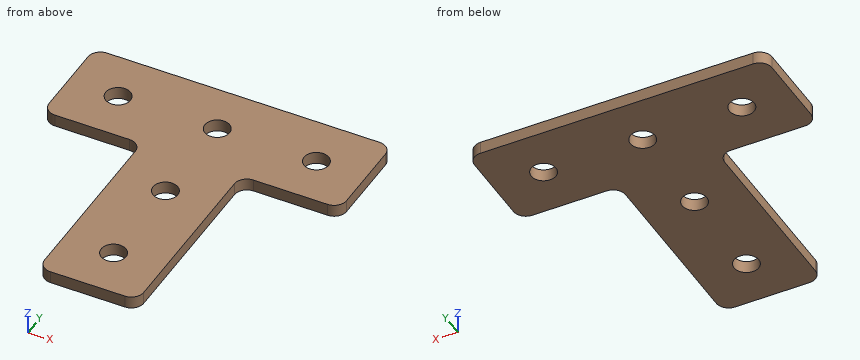
Autodesk Inventor part; units mm, degrees
ref_plane "YZ Plane" through (0, 0, 0) normal (1, 0, 0) x (0, 1, 0)
ref_plane "XZ Plane" through (0, 0, 0) normal (0, 1, 0) x (-1, 0, 0)
ref_plane "XY Plane" through (0, 0, 0) normal (0, 0, 1) x (1, 0, 0)
sketch "Sketch1" plane through (0, 0, 0) normal (0, 0, 1) x (1, 0, 0)
  line L0 (-18.0361, 37.9933) -> (2.0277, 37.9933)
  line L1 (6.0832, 12.5933) -> (6.0832, -38.2067)
  line L2 (6.0832, -38.2067) -> (-19.3168, -38.2067)
  line L3 (-19.3168, -38.2067) -> (-19.3168, 12.5933)
  line L4 (-44.7168, 37.9933) -> (31.4832, 37.9933)
  line L5 (31.4832, 37.9933) -> (31.4832, 12.5933)
  line L6 (-44.7168, 12.5933) -> (-44.7168, 37.9933)
  line L7 (31.4832, 12.5933) -> (6.0832, 12.5933)
  line L8 (-19.3168, 12.5933) -> (-44.7168, 12.5933)
  point P0 (0, 0)
  dimension "d0" = 76.2
  dimension "d1" = 25.4
  dimension "d2" = 25.4
  dimension "d3" = 25.4
  dimension "d4" = 50.8
  dimension "d5" = 25.4
extrude "Extrusion1" add sketch "Sketch1" along normal blind 3.175
fillet "Fillet1" radius 3.175 3 edges at (-44.7168, 12.5933, 1.5875) (-19.3168, 12.5933, 1.5875) (-19.3168, -38.2067, 1.5875)
fillet "Fillet2" radius 3.175 1 edges at (6.0832, -38.2067, 1.5875)
fillet "Fillet3" radius 3.175 3 edges at (6.0832, 12.5933, 1.5875) (31.4832, 12.5933, 1.5875) (31.4832, 37.9933, 1.5875)
fillet "Fillet4" radius 3.175 1 edges at (-44.7168, 37.9933, 1.5875)
sketch "Sketch2" plane through (0, 0, 3.175) normal (0, 0, 1) x (1, 0, 0)
  line L0 (31.4832, 15.7683) -> (31.4832, 34.8183)
  line L1 (31.4832, 25.2933) -> (-44.7168, 25.2933) construction
  line L2 (-44.7168, 34.8183) -> (-44.7168, 15.7683)
  line L3 (28.3082, 37.9933) -> (-41.5418, 37.9933)
  line L4 (-6.6168, 37.9933) -> (-6.6168, -38.2067) construction
  line L5 (-16.1418, -38.2067) -> (2.9082, -38.2067)
  circle A0 centre (18.7832, 25.2933) radius 3.175
  circle A1 centre (-6.6168, 25.2933) radius 3.175
  circle A2 centre (-32.0168, 25.2933) radius 3.175
  circle A3 centre (-6.6168, -0.1067) radius 3.175
  circle A4 centre (-6.6168, -25.5067) radius 3.175
  point P0 (0, 0)
  dimension "d12" = 6.35
  dimension "d13" = 12.7
  dimension "d16" = 25.4
  dimension "d23" = 25.4
extrude "Extrusion2" cut sketch "Sketch2" against normal through all
properties part number "Frame T Gussets"
The listing builds one solid part. Answer for the finished solid, in the listing's coordinates (mm). Coordinates: 2 decimals unless noted, no trailing zeros. Write each loop counter-clockwise with the first axis right and the second up, starting at its lowest first coordinate (ties: lowest second). Pieces come first, ordered by that corner, then holes. Notation, with made-up numbers: M -12,16 L 47,16 A33 ccw 47,51 Z; hole C 53,8 d1. An arc over 180 degrees is marked long. Use a Markdown table: item, result. Add a question column.
1. Given P1, Ø1.6, axis at y = -3.5, z = 2, coming from the +X side; P2, Ø8.5, axis at x = -6.62, y = -0.11, coming from the -Z side; P3, Ø1.6, axis at x = -34.5, z = 2, coming from the -Y side, each flat-ended and moving along its own axis, determine where each tip first touches the part or whether it passes through.
2. Section A-A (x = 11.5) is taken. Give the vertices of the cut face in (y, z) (3 decimals), plus the area to 3 significant figures.
3. Section B-B (y = -6) is taken. Give the vertices of the cut face in (x, z) (3 decimals).
4. Straight lines are drawn through the part: line 1 along X through (y, z) = (27, 1.1); line 2 along X through (y, z) = (7.5, 1.3); line 3 along Y through (x, z) = (11, 0.55). For each, find the intervals that lie inside material, in ascending order. Write a range as [from, to].
5. Section C-C (z = 1.3) is taken. Give the vertices of the cut face in (x, y) (3 decimals), plus the area to 3 significant figures.
Data:
| question | item | result |
|---|---|---|
| 1 | P1 | stops at x = 6.08 |
| 1 | P2 | stops at z = 0 |
| 1 | P3 | stops at y = 12.59 |
| 2 | outline | M 12.593,0 L 37.993,0 L 37.993,3.175 L 12.593,3.175 Z |
| 2 | area | 80.6 mm2 |
| 3 | outline | M -19.317,0 L 6.083,0 L 6.083,3.175 L -19.317,3.175 Z |
| 4 | line 1 | x = [-44.72, -34.69], [-29.34, -9.29], [-3.94, 16.11], [21.46, 31.48] |
| 4 | line 2 | x = [-19.32, 6.08] |
| 4 | line 3 | y = [12.59, 37.99] |
| 5 | outline | M -44.717,15.768 A3.175 ccw -41.542,12.593 L -22.492,12.593 A3.175 cw -19.317,9.418 L -19.317,-35.032 A3.175 ccw -16.142,-38.207 L 2.908,-38.207 A3.175 ccw 6.083,-35.032 L 6.083,9.418 A3.175 cw 9.258,12.593 L 28.308,12.593 A3.175 ccw 31.483,15.768 L 31.483,34.818 A3.175 ccw 28.308,37.993 L -41.542,37.993 A3.175 ccw -44.717,34.818 Z; hole C -32.017,25.293 d6.35; hole C -6.617,-25.507 d6.35; hole C -6.617,-0.107 d6.35; hole C -6.617,25.293 d6.35; hole C 18.783,25.293 d6.35 |
| 5 | area | 3,060 mm2 |
